```python
from build123d import *

# Parameters (mm, degrees)
SKETCH_1_R          = 19.5
EXTRUDE_1_DEPTH     = 32
SKETCH_2_R          = 7.88
EXTRUDE_2_DEPTH     = 5
CUT_EXTRUDE_1_REACH = 48.147
SKETCH_3_R          = 3
SKETCH_4_W          = 1
SKETCH_4_H          = 15
EXTRUDE_3_DEPTH     = 9.5
SKETCH_6_W          = 1
SKETCH_6_H          = 15
EXTRUDE_4_DEPTH     = 10
SKETCH_7_W          = 4
SKETCH_7_H          = 10
CUT_EXTRUDE_2_DEPTH = 10


with BuildPart() as part:
    # 草图1 → 凸台-拉伸1 (new body)
    with BuildSketch(Plane(origin=(0, 0, 0), x_dir=(0, 0, -1), z_dir=(1, 0, 0))):
        Circle(SKETCH_1_R)
    extrude(amount=EXTRUDE_1_DEPTH)

    # 草图2 → 凸台-拉伸2 (add)
    with BuildSketch(Plane(origin=(32, 0, 0), x_dir=(0, 0, -1), z_dir=(1, 0, 0))):
        Circle(SKETCH_2_R)
    extrude(amount=EXTRUDE_2_DEPTH)

    # 草图3 → 切除-拉伸1 (cut, up to next)
    with BuildSketch(Plane(origin=(37, 0, 0), x_dir=(0, 0, -1), z_dir=(1, 0, 0)), mode=Mode.PRIVATE) as cut_extrude_1_sk1:
        Circle(SKETCH_3_R)
    cut_extrude_1_tool1 = extrude(cut_extrude_1_sk1.sketch, amount=-CUT_EXTRUDE_1_REACH, mode=Mode.PRIVATE) & part.part
    add(cut_extrude_1_tool1.solids().sort_by_distance((37, 0, 0))[0], mode=Mode.SUBTRACT)

    # 草图4 → 凸台-拉伸3 (add)
    with BuildSketch(Plane(origin=(32, 0, 0), x_dir=(0, 0, -1), z_dir=(1, 0, 0))):
        with Locations((17.5, 0)):
            Rectangle(SKETCH_4_W, SKETCH_4_H)
    extrude_3 = extrude(amount=EXTRUDE_3_DEPTH)

    # 草图6 → 凸台-拉伸4 (add)
    with BuildSketch(Plane(origin=(0, 0, -18), x_dir=(-1, 0, 0), z_dir=(0, 0, -1))):
        with Locations((-41, 0)):
            Rectangle(SKETCH_6_W, SKETCH_6_H)
    extrude_4 = extrude(amount=EXTRUDE_4_DEPTH)

    # 草图7 → 切除-拉伸2 (cut)
    with BuildSketch(Plane(origin=(41.5, 0, 0), x_dir=(0, 0, -1), z_dir=(1, 0, 0))):
        with Locations((24, 0)):
            Rectangle(SKETCH_7_W, SKETCH_7_H)
    cut_extrude_2 = extrude(amount=-CUT_EXTRUDE_2_DEPTH, mode=Mode.SUBTRACT)

    # 镜向1: 凸台-拉伸3, 凸台-拉伸4, 切除-拉伸2 across plane
    add(extrude_3.mirror(Plane.XY))
    add(extrude_4.mirror(Plane.XY))
    add(cut_extrude_2.mirror(Plane.XY), mode=Mode.SUBTRACT)


solid = part.part
```
Geometry: final body of the model. Coordinates: model frame, mm. A direction names the side the tool comes from. Round coordinates to 2 decimals unless told otherwise and drop trailing zeros. Order: outer loops, then holes, each group sorted by start corner. A loop starts at its lowest first (then second) coordinate and runs counter-clockwise, first axis right, second up. Notation, with made-up numbers: (69.5, -22.5) - (103.5, -22.5) arc R32 cw to (103.5, 7.5) - close; hole circle Ø2 at (46.25, 72.5). An arc over 180 degrees is marked (long way). Write item = value, one per line. Start each with the question number.
Q1. Pin query (flat end, axial travel): pin 1 (1.1 mm diameter, centred on x = 41, z = -24, fed in from -Y); pin 2 (5 mm diameter, centred on x = 39, z = -24.5, fed in from +Y); pin 3 (5 mm diameter, centred on x = 36.5, z = 22, fed in from +Y); pin 4 (3 mm diameter, centred on y = 14.5, z = 10.5, fed in from +X). Return the tip coordinate at first contact, or that it passes through.
Q2. Access query for faces 4 (the flat face through (37, 0, -17)), 5 (the flat face through (41, -7.5, 20)), 6 (the flat face through (32, 0, -19)). Directions: +Z, -Z, +X, -X, +Y, -Y. A direction counts if a zero-diameter tool reaches every point of the face in a straight line with its end or side. Return the directions, or none.
Q3. Ray query, line 1 (Y direction, x = 9, z = 0); line 2 (X direction, y = -7.5, z = 3.5); line 3 (X direction, y = 3.5, z = 5). Return the intervals inside material, ascending. Write a range as from..to.
Q4. Cut plane D-D on y = 10.5. Return the cut outline in (x, z).
Q5. Cut plane B-B on z = 0. Return the cut outline in (x, y).
Q6. Cut plane C-C on x = 9. Return the cut outline in (y, z), and give its area (3 significant figures).
Q7. Pull-direction query (Z, two-part tool) for faces 1 (the flat face through (37, 0.1, -3.4)), 2 (the flat face through (36, 0, 18)), 3 (the flat face through (32, 0, 19)); classes: +Z half, -Z half, draft (parallel to the pull), parting line (faces both ways), or undercut.
Q8. Cut plane A-A on y = 0. Give the number of separate pieces and of enclosed holes in the cut face, and give its area (3 significant figures).
Outcome:
q1.pin_1 = -7.5
q1.pin_2 = 7.5
q1.pin_3 = through
q1.pin_4 = 32
q2.face_4 = +X, +Y, -Y
q2.face_5 = +Z, +X, -Y
q2.face_6 = -Z, +Y, -Y
q3.line_1 = -19.5..-3, 3..19.5
q3.line_2 = 0..32
q3.line_3 = 0..37
q4.outline = (0, -16.43) - (32, -16.43) - (32, 16.43) - (0, 16.43) - close
q5.outline = (0, -19.5) - (32, -19.5) - (32, -7.88) - (37, -7.88) - (37, -3) - (0, -3) - close; (0, 3) - (37, 3) - (37, 7.88) - (32, 7.88) - (32, 19.5) - (0, 19.5) - close
q6.outline = circle Ø39 at (0, 0); hole circle Ø6 at (0, 0)
q6.area = 1,170 mm^2
q7.face_1 = undercut
q7.face_2 = +Z half
q7.face_3 = draft
q8.separate_pieces = 4
q8.enclosed_holes = 0
q8.area = 1,140 mm^2
